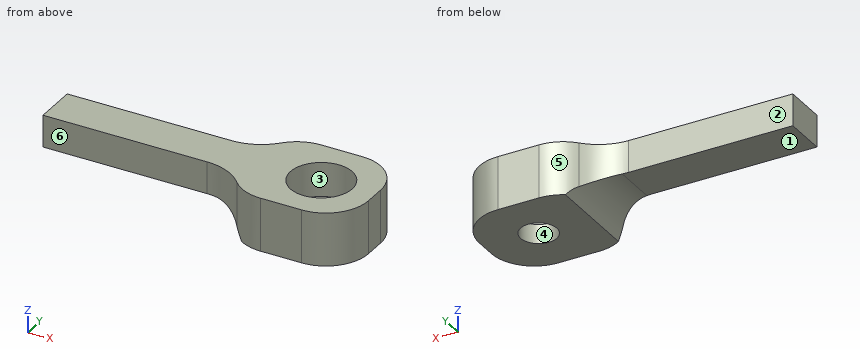
from build123d import *

# Parameters (mm, degrees)
SKETCH1_W           = 38.1
SKETCH1_H           = 12.7
BOSS_EXTRUDE1_DEPTH = 6.35
SKETCH2_R           = 2.159
CUT_EXTRUDE1_DEPTH  = 33.995567884
SKETCH3_R           = 3.683
CUT_EXTRUDE2_DEPTH  = 4.064
SKETCH5_W           = 25.4
SKETCH5_H           = 3.81
CUT_EXTRUDE3_DEPTH  = 33.995567884
SKETCH6_W           = 25.4
SKETCH6_H           = 2.54
CUT_EXTRUDE4_DEPTH  = 34.577032329
FILLET3_R           = 6.35
FILLET4_R           = 5.08


with BuildPart() as part:
    # Sketch1 → Boss-Extrude1 (new body)
    with BuildSketch(Plane.XY):
        with Locations((-12.7, 0)):
            Rectangle(SKETCH1_W, SKETCH1_H)
    extrude(amount=BOSS_EXTRUDE1_DEPTH)

    # Sketch2 → Cut-Extrude1 (cut, through all)
    with BuildSketch(Plane.XY.offset(6.35)):
        Circle(SKETCH2_R)
    extrude(amount=-CUT_EXTRUDE1_DEPTH, mode=Mode.SUBTRACT)

    # Sketch3 → Cut-Extrude2 (cut)
    with BuildSketch(Plane.XY.offset(6.35)):
        Circle(SKETCH3_R)
    extrude(amount=-CUT_EXTRUDE2_DEPTH, mode=Mode.SUBTRACT)

    # Sketch5 → Cut-Extrude3 (cut, through all)
    with BuildSketch(Plane.XY.offset(6.35)):
        with Locations((-19.05, 4.445)):
            Rectangle(SKETCH5_W, SKETCH5_H)
        with Locations((-19.05, -4.445)):
            Rectangle(SKETCH5_W, SKETCH5_H)
    extrude(amount=-CUT_EXTRUDE3_DEPTH, mode=Mode.SUBTRACT)

    # Sketch6 → Cut-Extrude4 (cut, through all)
    with BuildSketch(Plane(origin=(0, 2.54, 0), x_dir=(1, 0, 0), z_dir=(0, 1, 0))):
        with Locations((-19.05, -1.27)):
            Rectangle(SKETCH6_W, SKETCH6_H)
    extrude(amount=-CUT_EXTRUDE4_DEPTH, mode=Mode.SUBTRACT)

    # Fillet3
    # the kernel refuses this fillet: 6.35 mm, written as the material it adds along each edge
    with BuildSketch(Plane(origin=(-6.35, -2.54, 6.35), x_dir=(-1, 0, 0), z_dir=(0, 0, -1))) as fillet3_piece_1:
        with BuildLine():
            CenterArc((5.819871133, -6.35), FILLET3_R, 90, 66.421821522)
            Line((0, -3.81), (-0.116397423, -3.7592))
            ThreePointArc((-0.116397423, -3.7592), (-0.127, -1.905), (-0.127, 0))
            Line((-0.127, 0), (0, 0.127))
            Line((0, 0.127), (5.819871133, 0.127))
            Line((5.819871133, 0.127), (5.819871133, 0))
        make_face()
    extrude(amount=3.81)
    with BuildSketch(Plane(origin=(-6.35, 2.54, 2.54), x_dir=(-1, 0, 0), z_dir=(0, -1, 0))) as fillet3_piece_2:
        with BuildLine():
            CenterArc((5.08, 6.35), FILLET3_R, 216.869897646, 53.130102354)
            Line((0, 2.54), (-0.1016, 2.4638))
            ThreePointArc((-0.1016, 2.4638), (-0.127, 1.27), (-0.127, 0))
            Line((-0.127, 0), (0, -0.127))
            Line((0, -0.127), (5.08, -0.127))
            Line((5.08, -0.127), (5.08, 0))
        make_face()
    extrude(amount=5.08)
    with BuildSketch(Plane(origin=(-6.35, 2.54, 6.35), x_dir=(-1, 0, 0), z_dir=(0, 0, -1))) as fillet3_piece_3:
        with BuildLine():
            CenterArc((5.819871133, 6.35), FILLET3_R, 203.578178478, 66.421821522)
            Line((0, 3.81), (-0.116397423, 3.7592))
            ThreePointArc((-0.116397423, 3.7592), (-0.127, 1.905), (-0.127, 0))
            Line((-0.127, 0), (0, -0.127))
            Line((0, -0.127), (5.819871133, -0.127))
            Line((5.819871133, -0.127), (5.819871133, 0))
        make_face()
    extrude(amount=3.81)
    with BuildSketch(Plane(origin=(-6.35, 2.54, 2.54), x_dir=(-1, 0, 0), z_dir=(0, -1, 0))) as fillet3_piece_4a_section:
        with BuildLine():
            CenterArc((5.08, 6.35), FILLET3_R, 216.869897646, 53.130102354)
            Line((0, 2.54), (-0.1016, 2.4638))
            ThreePointArc((-0.1016, 2.4638), (-0.127, 1.27), (-0.127, 0))
            Line((-0.127, 0), (0, -0.127))
            Line((0, -0.127), (5.08, -0.127))
            Line((5.08, -0.127), (5.08, 0))
        make_face()
    fillet3_piece_4a = extrude(amount=17.78, mode=Mode.PRIVATE)
    fillet3_piece_4a = split(fillet3_piece_4a, bisect_by=Plane(origin=(-7.657359662, -6.35, 1.889832946), z_dir=(0, 1, 0)), keep=Keep.TOP, mode=Mode.PRIVATE)
    fillet3_piece_4a = split(fillet3_piece_4a, bisect_by=Plane(origin=(-7.657359662, -2.54, 1.889832946), z_dir=(0, -1, 0)), keep=Keep.TOP, mode=Mode.PRIVATE)
    with BuildSketch(Plane(origin=(-6.35, -2.54, 6.35), x_dir=(-1, 0, 0), z_dir=(0, 0, -1))) as fillet3_piece_4b_section:
        with BuildLine():
            CenterArc((5.819871133, -6.35), FILLET3_R, 90, 66.421821522)
            Line((0, -3.81), (-0.116397423, -3.7592))
            ThreePointArc((-0.116397423, -3.7592), (-0.127, -1.905), (-0.127, 0))
            Line((-0.127, 0), (0, 0.127))
            Line((0, 0.127), (5.819871133, 0.127))
            Line((5.819871133, 0.127), (5.819871133, 0))
        make_face()
    fillet3_piece_4b = extrude(amount=18.359677831, mode=Mode.PRIVATE)
    fillet3_piece_4b = split(fillet3_piece_4b, bisect_by=Plane(origin=(-7.767240906, -3.525286877, 2.54), z_dir=(0, 0, -1)), keep=Keep.TOP, mode=Mode.PRIVATE)
    fillet3_piece_4b = split(fillet3_piece_4b, bisect_by=Plane(origin=(-7.767240906, -3.525286877, 0), z_dir=(0, 0, 1)), keep=Keep.TOP, mode=Mode.PRIVATE)
    fillet3_piece_4 = fillet3_piece_4a & fillet3_piece_4b
    add(fillet3_piece_4)
    with BuildSketch(Plane(origin=(-6.35, 2.54, 6.35), x_dir=(-1, 0, 0), z_dir=(0, 0, -1))) as fillet3_piece_5a_section:
        with BuildLine():
            CenterArc((5.819871133, 6.35), FILLET3_R, 203.578178478, 66.421821522)
            Line((0, 3.81), (-0.116397423, 3.7592))
            ThreePointArc((-0.116397423, 3.7592), (-0.127, 1.905), (-0.127, 0))
            Line((-0.127, 0), (0, -0.127))
            Line((0, -0.127), (5.819871133, -0.127))
            Line((5.819871133, -0.127), (5.819871133, 0))
        make_face()
    fillet3_piece_5a = extrude(amount=18.359677831, mode=Mode.PRIVATE)
    fillet3_piece_5a = split(fillet3_piece_5a, bisect_by=Plane(origin=(-7.767240906, 3.525286877, 2.54), z_dir=(0, 0, -1)), keep=Keep.TOP, mode=Mode.PRIVATE)
    fillet3_piece_5a = split(fillet3_piece_5a, bisect_by=Plane(origin=(-7.767240906, 3.525286877, 0), z_dir=(0, 0, 1)), keep=Keep.TOP, mode=Mode.PRIVATE)
    with BuildSketch(Plane(origin=(-6.35, 15.24, 2.54), x_dir=(-1, 0, 0), z_dir=(0, -1, 0))) as fillet3_piece_5b_section:
        with BuildLine():
            CenterArc((5.08, 6.35), FILLET3_R, 216.869897646, 53.130102354)
            Line((0, 2.54), (-0.1016, 2.4638))
            ThreePointArc((-0.1016, 2.4638), (-0.127, 1.27), (-0.127, 0))
            Line((-0.127, 0), (0, -0.127))
            Line((0, -0.127), (5.08, -0.127))
            Line((5.08, -0.127), (5.08, 0))
        make_face()
    fillet3_piece_5b = extrude(amount=17.78, mode=Mode.PRIVATE)
    fillet3_piece_5b = split(fillet3_piece_5b, bisect_by=Plane(origin=(-7.657359662, 6.35, 1.889832946), z_dir=(0, -1, 0)), keep=Keep.TOP, mode=Mode.PRIVATE)
    fillet3_piece_5b = split(fillet3_piece_5b, bisect_by=Plane(origin=(-7.657359662, 2.54, 1.889832946), z_dir=(0, 1, 0)), keep=Keep.TOP, mode=Mode.PRIVATE)
    fillet3_piece_5 = fillet3_piece_5a & fillet3_piece_5b
    add(fillet3_piece_5)

    # Fillet4
    fillet4_edges = [part.edges().sort_by_distance(p)[0] for p in [
        (-6.35, 6.35, 3.175),
        (-6.35, -6.35, 3.175),
        (6.35, -6.35, 3.175),
        (6.35, 6.35, 3.175),
    ]]
    fillet(fillet4_edges, radius=FILLET4_R)


solid = part.part
Build history of the part. All positions in model axes, mm. Face numbers are marked on the shaded views. A direction names the side the tool comes from. Give positions to 0.01 mm unless a question says otherwise; leave off trailing zeros. Write each loop counter-clockwise with the first axis right and the second up, starting at its lowest first coordinate (ties: lowest second). Pieces come first, ordered by that corner, then holes. Notation, with made-up numbers: (-3, 59) - (7, 59) arc R24 ccw to (7, 82) - close; hole circle Ø3 at (66.25, -33.5). An arc over 180 degrees is marked (long way). Use one line per item in the form item = value. Start each with the question number.
1. Band-saw the part on D-D on y = 1.75. Write the cut outline in (x, z), plus the area to 3 significant figures.
2. Drop flat-ended pins along their axis: pin 1 Ø1.5 at (x, y) = (-12, 1.5) entering from -Z; pin 2 Ø6.5 at (x, y) = (0, 0) entering from +Z; pin 3 Ø3 at (x, z) = (-24, 3.5) entering from +Y. Give the stop position or say it passes through.
3. Band-saw the part on C-C on y = 0. Write the cut outline in (x, z).
4. Probe line 1 (Y direction, x = 0, z = 6); line 2 (Y direction, x = 0, z = 1.3); line 3 (Z direction, x = -12, y = -1.75). List the from-to ranges inside material, lowest first. Write a range as [from, to].
5. Band-saw the part on A-A on z = 5. Write the cut outline in (x, y).
6. 3-axis set-ups, long thin cutter, end or side, ignore diameter. For the marked faces 1, 2 and 3: which of +Z, -Z, +X, -X, +Y, -Y reach the whole face in a straight line?
7. Band-saw the part on B-B on x = 0. Write the cut outline in (y, z).
8. Two-plate mould, pull along Y, no slides. Class the marked faces 4, 5 and 6: released by +Y, released by -Y, zero draft, split by the parting line, or undercut.
Conclusion:
q1.outline = (-31.75, 2.54) - (-11.43, 2.54) arc R6.35 cw to (-6.35, 0) - (-1.26, 0) - (-1.26, 2.29) - (-3.24, 2.29) - (-3.24, 6.35) - (-31.75, 6.35) - close; (1.26, 0) - (6.33, 0) - (6.33, 6.35) - (3.24, 6.35) - (3.24, 2.29) - (1.26, 2.29) - close
q1.area = 149 mm²
q2.pin_1 = 2.54
q2.pin_2 = 2.29
q2.pin_3 = 2.54
q3.outline = (-31.75, 2.54) - (-11.43, 2.54) arc R6.35 cw to (-6.35, 0) - (-2.16, 0) - (-2.16, 2.29) - (-3.68, 2.29) - (-3.68, 6.35) - (-31.75, 6.35) - close; (2.16, 0) - (6.35, 0) - (6.35, 6.35) - (3.68, 6.35) - (3.68, 2.29) - (2.16, 2.29) - close
q4.line_1 = [-6.35, -3.68], [3.68, 6.35]
q4.line_2 = [-6.35, -2.16], [2.16, 6.35]
q4.line_3 = [2.54, 6.35]
q5.outline = (-31.75, -2.54) - (-12.17, -2.54) arc R6.35 cw to (-7.44, -4.66) arc R5.08 ccw to (-3.65, -6.35) - (1.27, -6.35) arc R5.08 ccw to (6.35, -1.27) - (6.35, 1.27) arc R5.08 ccw to (1.27, 6.35) - (-3.65, 6.35) arc R5.08 ccw to (-7.44, 4.66) arc R6.35 cw to (-12.17, 2.54) - (-31.75, 2.54) - close; hole circle Ø7.37 at (0, 0)
q6.face_1 = -Z, -X, +Y, -Y
q6.face_2 = +Z, -Z, -X, +Y
q6.face_3 = +Z
q7.outline = (-6.35, 0) - (-2.16, 0) - (-2.16, 2.29) - (-3.68, 2.29) - (-3.68, 6.35) - (-6.35, 6.35) - close; (2.16, 0) - (6.35, 0) - (6.35, 6.35) - (3.68, 6.35) - (3.68, 2.29) - (2.16, 2.29) - close
q8.face_4 = undercut
q8.face_5 = released by +Y
q8.face_6 = released by -Y
